Answer from the drawing. Dimensions are ordinates in mm from the lowest x, y and z of the part. Coordinates: 2 decimals unless noted, no trailing zeros. Write each loop counter-clockwise with the first axis right and the second up, starting at its lowest first coordinate (ties: lowest second). Pieces come first, ordered by that corner, then holes. Notation, with made-up numbers: (-1.5, 44) -> (46.5, 44) arc R21 cw to (46.5, 77) -> close; hole circle Ø7 at (80.25, 42). An arc over 180 degrees is marked (long way). Return JSON: item names as keys, results as strings.
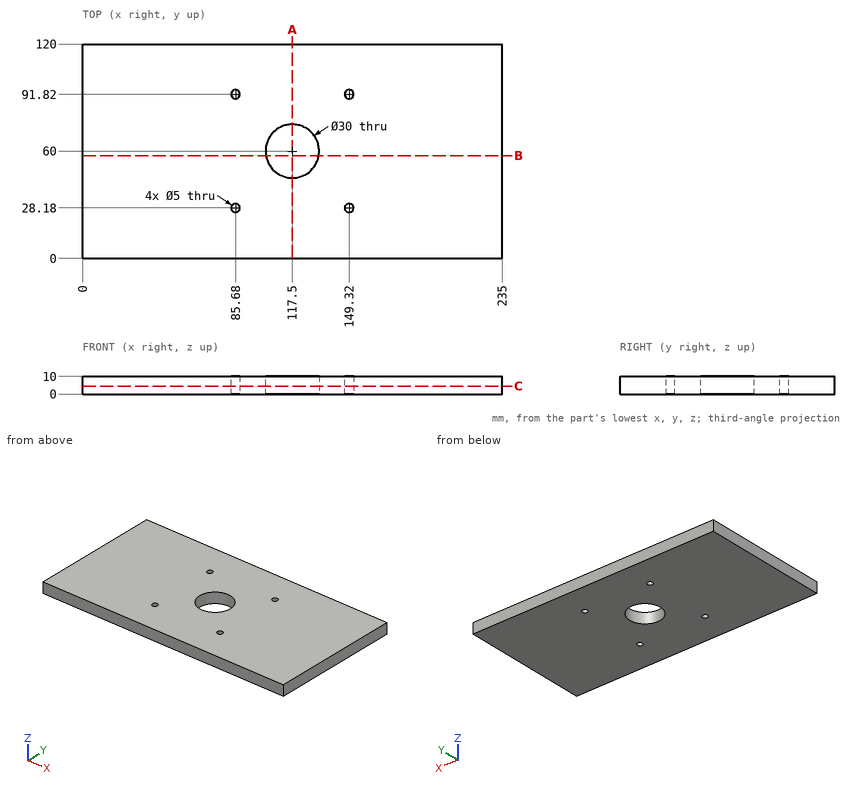
1. Consider L1, parallel to X at y = 91.5, z = 6.25; L2, parallel to Y at x = 117.5, z = 8; L3, parallel to Y at x = 84.5, z = 2. Determine where each line is inside the solid, lowest interval first.
Taken from the geometry:
{"L1": "x = 0 to 83.2, 88.16 to 146.84, 151.8 to 235", "L2": "y = 0 to 45, 75 to 120", "L3": "y = 0 to 25.98, 30.38 to 89.62, 94.02 to 120"}
2. The part is cut by section A-A (x = 117.5). Determine the outline of the cut face in (y, z), then the cut area to 3 significant figures.
Taken from the geometry:
{"outline": "(0, 0) -> (45, 0) -> (45, 10) -> (0, 10) -> close; (75, 0) -> (120, 0) -> (120, 10) -> (75, 10) -> close", "area": "900 mm2"}
3. The part is cut by section B-B (y = 57.5). Determine the outline of the cut face in (x, z).
Taken from the geometry:
{"outline": "(0, 0) -> (102.71, 0) -> (102.71, 10) -> (0, 10) -> close; (132.29, 0) -> (235, 0) -> (235, 10) -> (132.29, 10) -> close"}
4. The part is cut by section C-C (z = 4.5). Determine the outline of the cut face in (x, y).
Taken from the geometry:
{"outline": "(0, 0) -> (235, 0) -> (235, 120) -> (0, 120) -> close; hole circle Ø5 at (85.68, 28.18); hole circle Ø5 at (85.68, 91.82); hole circle Ø30 at (117.5, 60); hole circle Ø5 at (149.32, 28.18); hole circle Ø5 at (149.32, 91.82)"}
